```python
from build123d import *

# Parameters (mm, degrees)
SKETCH1_W                                      = 45
SKETCH1_H                                      = 73
SKETCH1_R                                      = 20.25
BOSS_EXTRUDE1_DEPTH                            = 5
CHAMFER1_SIZE                                  = 4
SKETCH2_W                                      = 45
SKETCH2_H                                      = 17
BOSS_EXTRUDE2_DEPTH                            = 32.5
CBORE_SLOT_FOR_M6_HEX_SOCKET_HEAD_CAP_SC_DEPTH = 17
CBORE_START                                    = 10.5
CBORE_SLOT_FOR_M6_HEX_SOCKET_HEAD_CA_3_DEPTH   = 6.5


# Read off the part's stored shape, not the designer's step: CBORE SLOT for M6 Hex Socket Head Cap Screw1
with BuildPart() as part:
    # Sketch1 → Boss-Extrude1 (new body)
    with BuildSketch(Plane(origin=(0, 0, 0), x_dir=(0, 0, -1), z_dir=(1, 0, 0))):
        with Locations((0, 36.5)):
            Rectangle(SKETCH1_W, SKETCH1_H)
        with Locations((0, 47.5)):
            Circle(SKETCH1_R, mode=Mode.SUBTRACT)
    extrude(amount=BOSS_EXTRUDE1_DEPTH)

    # Chamfer1
    chamfer1_edges = [part.edges().sort_by_distance(p)[0] for p in [
        (2.5, 73, 22.5),
        (2.5, 73, -22.5),
    ]]
    chamfer(chamfer1_edges, length=CHAMFER1_SIZE)

    # Sketch2 → Boss-Extrude2 (add)
    with BuildSketch(Plane.ZY):
        with Locations((0, 8.5)):
            Rectangle(SKETCH2_W, SKETCH2_H)
    extrude(amount=BOSS_EXTRUDE2_DEPTH)

    # CBORE SLOT for M6 Hex Socket Head Ca 2 → CBORE SLOT for M6 Hex Socket Head Cap Screw1 (cut)
    with BuildSketch(Plane(origin=(0, 0, 0), x_dir=(1, 0, 0), z_dir=(0, 1, 0))):
        with BuildLine():
            Line((-24.2, -15.8), (-5.8, -15.8))
            ThreePointArc((-5.8, -15.8), (-2.5, -12.5), (-5.8, -9.2))
            Line((-5.8, -9.2), (-24.2, -9.2))
            ThreePointArc((-24.2, -9.2), (-27.5, -12.5), (-24.2, -15.8))
        make_face()
        with BuildLine():
            Line((-24.2, 9.2), (-5.8, 9.2))
            ThreePointArc((-5.8, 9.2), (-2.5, 12.5), (-5.8, 15.8))
            Line((-5.8, 15.8), (-24.2, 15.8))
            ThreePointArc((-24.2, 15.8), (-27.5, 12.5), (-24.2, 9.2))
        make_face()
    extrude(amount=CBORE_SLOT_FOR_M6_HEX_SOCKET_HEAD_CAP_SC_DEPTH, mode=Mode.SUBTRACT)

    # CBORE SLOT for M6 Hex Socket Head Ca 3 o → CBORE SLOT for M6 Hex Socket Head Ca 3 (cut)
    # profile 1 of 2: a face of its own
    with BuildSketch(Plane(origin=(0, 0, 0), x_dir=(1, 0, 0), z_dir=(0, 1, 0)).offset(CBORE_START)):
        with BuildLine():
            Line((-24.2, -18), (-5.8, -18))
            ThreePointArc((-5.8, -18), (-0.3, -12.5), (-5.8, -7))
            Line((-5.8, -7), (-24.2, -7))
            ThreePointArc((-24.2, -7), (-29.7, -12.5), (-24.2, -18))
        make_face()
        with BuildLine():
            ThreePointArc((-5.8, -9.2), (-2.5, -12.5), (-5.8, -15.8))
            Line((-5.8, -15.8), (-24.2, -15.8))
            ThreePointArc((-24.2, -15.8), (-27.5, -12.5), (-24.2, -9.2))
            Line((-24.2, -9.2), (-5.8, -9.2))
        make_face(mode=Mode.SUBTRACT)
    # profile 2 of 2: a face of its own
    with BuildSketch(Plane(origin=(0, 0, 0), x_dir=(1, 0, 0), z_dir=(0, 1, 0)).offset(CBORE_START)):
        with BuildLine():
            Line((-24.2, 7), (-5.8, 7))
            ThreePointArc((-5.8, 7), (-0.3, 12.5), (-5.8, 18))
            Line((-5.8, 18), (-24.2, 18))
            ThreePointArc((-24.2, 18), (-29.7, 12.5), (-24.2, 7))
        make_face()
        with BuildLine():
            ThreePointArc((-5.8, 15.8), (-2.5, 12.5), (-5.8, 9.2))
            Line((-5.8, 9.2), (-24.2, 9.2))
            ThreePointArc((-24.2, 9.2), (-27.5, 12.5), (-24.2, 15.8))
            Line((-24.2, 15.8), (-5.8, 15.8))
        make_face(mode=Mode.SUBTRACT)
    extrude(amount=CBORE_SLOT_FOR_M6_HEX_SOCKET_HEAD_CA_3_DEPTH, mode=Mode.SUBTRACT)


solid = part.part
```
For this review, take the finished solid that the model builds, in its own axes (mm). A direction names the side the tool comes from. Coordinates: 2 decimals unless noted, no trailing zeros. Loops run counter-clockwise (first coordinate to the right, second up) from the corner with the lowest first, then second, coordinate; pieces in that order, holes last. Notation, with made-up numbers: (72, 16) -> (108, 16) arc R10 cw to (108, 28) -> close; hole circle Ø4 at (-27, 15.25). An arc over 180 degrees is marked (long way). Return JSON: item names as keys, results as strings. Group by question number.
(1) Consider section B-B, the plane y = 47.5. Give the boundary of the cut face in (x, z).
(2) Tool access review of faces 4 (the flat face through (-15, 14, 18)), 5 (the flat face through (-16, 17, 0)), 6 (the flat face through (-15, 5, 9.2)): name each direction out of +Z, -Z, +X, -X, +Y, -Y from which nothing blocks a thin tool from reaching the whole face with its end or side.
(3) For pin 1 Ø4 at (x, z) = (-10.5, 16.5) entering from +Y; pin 2 Ø22.5 at (y, z) = (37.5, 5.5) entering from -X, all flat-tipped, find the tip position at first contact; note any pin that passes through.
(4) Consider section C-C, the plane x = 1. Give the boundary of the cut face in (y, z).
(5) Mouldability with a two-part tool opening along Z and no side actions: class faces 1 (the flat face through (0, 27, 0)), 2 (the flat face through (-11, 16, -22.5)), 3 (the flat face through (-15, 14, -18)) as pulls with the +Z half, pulls with the -Z half, needs draft (parallel to the pull), parting line crosses it, or undercut.
(6) Consider section A-A, the plane z = 0. Give the boundary of the cut face in (x, y), plus the area to 3 significant figures.
(7) Consider section D-D, the plane x = -16.5. Give the boundary of the cut face in (y, z).
(8) To check wall thickness, follow L1, parallel to Y at x = 2.1, z = 0; L2, parallel to Y at x = -3, z = 9; L3, parallel to X at y = 37.5, z = 20.5. State the ranges of each line that lie inside material, in increasing order.
Results below:
{
 "1": {"outline": "(0, -22.5) -> (5, -22.5) -> (5, -20.25) -> (0, -20.25) -> close; (0, 20.25) -> (5, 20.25) -> (5, 22.5) -> (0, 22.5) -> close"},
 "2": {"face 4": "+Y", "face 5": "+Z, -Z, -X, +Y", "face 6": "+Y, -Y"},
 "3": {"pin 1": "stops at y = 17", "pin 2": "stops at x = 0"},
 "4": {"outline": "(0, -22.5) -> (69, -22.5) -> (73, -18.5) -> (73, 18.5) -> (69, 22.5) -> (0, 22.5) -> close; hole circle Ø40.5 at (47.5, 0)"},
 "5": {"face 1": "needs draft", "face 2": "pulls with the -Z half", "face 3": "undercut"},
 "6": {"outline": "(-32.5, 0) -> (5, 0) -> (5, 27.25) -> (0, 27.25) -> (0, 17) -> (-32.5, 17) -> close; (0, 67.75) -> (5, 67.75) -> (5, 73) -> (0, 73) -> close", "area": "715 mm2"},
 "7": {"outline": "(0, -22.5) -> (17, -22.5) -> (17, -18) -> (10.5, -18) -> (10.5, -15.8) -> (0, -15.8) -> close; (0, -9.2) -> (10.5, -9.2) -> (10.5, -7) -> (17, -7) -> (17, 7) -> (10.5, 7) -> (10.5, 9.2) -> (0, 9.2) -> close; (0, 15.8) -> (10.5, 15.8) -> (10.5, 18) -> (17, 18) -> (17, 22.5) -> (0, 22.5) -> close"},
 "8": {"L1": "y = 0 to 27.25, 67.75 to 73", "L2": "y = 0 to 10.5", "L3": "x = 0 to 5"}
}
